For this review, take the finished solid that the model builds, in its own axes (mm). Coordinates: 2 decimals unless noted, no trailing zeros. Write each loop counter-clockwise with the first axis right and the second up, starting at its lowest first coordinate (ties: lowest second). Pieces come first, ordered by that corner, then holes. Notation, with made-up numbers: M 17.25,-37.5 L 69.25,-37.5 A32 cw 69.25,-3.5 Z; hole C -24.75,-32 d1. An arc over 180 degrees is marked long. One line per question, with ' | ' between items.
from build123d import *

# Parameters (mm, degrees)
F1_DEPTH  = 5
F0_W      = 115
F0_H      = 3
F0_W_2    = 3
F0_H_2    = 115
F2_DEPTH  = 2
F3_R      = 2.5
F4_DEPTH  = 5
F5_W      = 149
F5_H      = 149
F6_DEPTH  = 35
F7_R      = 1.5
F8_DEPTH  = 35
F9_W      = 149
F9_H      = 50.5775869712
F10_DEPTH = 200
F12_DEPTH = 2
F13_SIZE  = 1.99999


# Not quite as in the source:
# - a fillet or chamfer is up to 0.001 mm smaller than in the source, because OpenCascade refuses the exact size


with BuildPart() as f1:
    # F0 (on Top) → F1 (new body)
    with BuildSketch(Plane.XY):
        Polygon((74.5, 74.5), (60.5, 74.5), (-60.5, 74.5), (-74.5, 74.5), (-74.5, 60.5), (-74.5, -60.5), (-74.5, -74.5), (-60.5, -74.5), (60.5, -74.5), (74.5, -74.5), (74.5, -60.5), (74.5, 60.5), align=None)
        Polygon((57.5, 60.5), (60.5, 60.5), (60.5, 57.5), (60.5, -57.5), (60.5, -60.5), (57.5, -60.5), (-57.5, -60.5), (-60.5, -60.5), (-60.5, -57.5), (-60.5, 57.5), (-60.5, 60.5), (-57.5, 60.5), align=None, mode=Mode.SUBTRACT)
    extrude(amount=F1_DEPTH)

    # F0 (on Top) → F2 (join)
    with BuildSketch(Plane.XY):
        with Locations((0, 59)):
            Rectangle(F0_W, F0_H)
        with Locations((59, 59)):
            Rectangle(F0_W_2, F0_H)
        with Locations((59, 0)):
            Rectangle(F0_W_2, F0_H_2)
        with Locations((59, -59)):
            Rectangle(F0_W_2, F0_H)
        with Locations((0, -59)):
            Rectangle(F0_W, F0_H)
        with Locations((-59, 0)):
            Rectangle(F0_W_2, F0_H_2)
        with Locations((-59, -59)):
            Rectangle(F0_W_2, F0_H)
        with Locations((-59, 59)):
            Rectangle(F0_W_2, F0_H)
    extrude(amount=F2_DEPTH)

    # F3 (on face) → F4 (cut, through all)
    with BuildSketch(Plane.XY.offset(5)):
        with Locations((42.5219088793, 68.0854469538)):
            Circle(F3_R)
    extrude(amount=-F4_DEPTH, mode=Mode.SUBTRACT)

    # F5 (on face) → F6 (join)
    with BuildSketch(Plane.XY.offset(5)):
        Rectangle(F5_W, F5_H)
        Polygon((-60.5, 71.5), (60.5, 71.5), (71.5, 71.5), (71.5, 60.5), (71.5, -60.5), (71.5, -71.5), (60.5, -71.5), (-60.5, -71.5), (-71.5, -71.5), (-71.5, -60.5), (-71.5, 60.5), (-71.5, 71.5), align=None, mode=Mode.SUBTRACT)
    extrude(amount=F6_DEPTH)

    # F7 (on face) → F8 (join)
    with BuildSketch(Plane.XY.offset(40)):
        with BuildLine():
            ThreePointArc((-71.5, 64.975068144), (-66.8161183572, 65.4466893403), (-64.6000009775, 69.6000009775))
            ThreePointArc((-64.6000009775, 69.6000009775), (-64.6946638756, 70.5683335217), (-64.975068144, 71.5))
            Line((-64.975068144, 71.5), (-71.5, 71.5))
            Line((-71.5, 71.5), (-71.5, 64.975068144))
        make_face()
        with Locations((-69.6000009775, 69.6000009775)):
            Circle(F7_R, mode=Mode.SUBTRACT)
        with BuildLine():
            Line((71.5, 71.5), (64.975068144, 71.5))
            ThreePointArc((64.975068144, 71.5), (66.0644670716, 66.0644670716), (71.5, 64.975068144))
            Line((71.5, 64.975068144), (71.5, 71.5))
        make_face()
        with Locations((69.6000009775, 69.6000009775)):
            Circle(F7_R, mode=Mode.SUBTRACT)
        with BuildLine():
            Line((71.5, -71.5), (71.5, -64.975068144))
            ThreePointArc((71.5, -64.975068144), (66.0644670716, -66.0644670716), (64.975068144, -71.5))
            Line((64.975068144, -71.5), (71.5, -71.5))
        make_face()
        with Locations((69.6000009775, -69.6000009775)):
            Circle(F7_R, mode=Mode.SUBTRACT)
        with BuildLine():
            ThreePointArc((-64.6000009775, -69.6000009775), (-66.8161183572, -65.4466893403), (-71.5, -64.975068144))
            Line((-71.5, -64.975068144), (-71.5, -71.5))
            Line((-71.5, -71.5), (-64.975068144, -71.5))
            ThreePointArc((-64.975068144, -71.5), (-64.6946638756, -70.5683335217), (-64.6000009775, -69.6000009775))
        make_face()
        with Locations((-69.6000009775, -69.6000009775)):
            Circle(F7_R, mode=Mode.SUBTRACT)
    extrude(amount=-F8_DEPTH)

    # F9 (on face) → F10 (cut)
    with BuildSketch(Plane.XZ.offset(74.5)):
        with Locations((0, 12.7112065144)):
            Rectangle(F9_W, F9_H)
    extrude(amount=-F10_DEPTH, mode=Mode.SUBTRACT)

    # F11 (on face) → F12 (join)
    with BuildSketch(Plane.XY.offset(40)):
        with BuildLine():
            ThreePointArc((-64.975068144, 71.5), (-64.6974956073, 68.6174323567), (-66.0644670716, 66.0644670716))
            Line((-66.0644670716, 66.0644670716), (66.0644670716, 66.0644670716))
            ThreePointArc((66.0644670716, 66.0644670716), (64.6974956073, 68.6174323567), (64.975068144, 71.5))
            Line((64.975068144, 71.5), (-64.975068144, 71.5))
        make_face()
        with BuildLine():
            ThreePointArc((71.5, 64.975068144), (68.6174323567, 64.6974956073), (66.0644670716, 66.0644670716))
            Line((66.0644670716, 66.0644670716), (66.0644670716, -66.0644670716))
            ThreePointArc((66.0644670716, -66.0644670716), (68.6174323567, -64.6974956073), (71.5, -64.975068144))
            Line((71.5, -64.975068144), (71.5, 64.975068144))
        make_face()
        with BuildLine():
            Line((66.0644670716, -66.0644670716), (-66.0644670716, -66.0644670716))
            ThreePointArc((-66.0644670716, -66.0644670716), (-64.6974956073, -68.6174323567), (-64.975068144, -71.5))
            Line((-64.975068144, -71.5), (64.975068144, -71.5))
            ThreePointArc((64.975068144, -71.5), (64.6974956073, -68.6174323567), (66.0644670716, -66.0644670716))
        make_face()
        with BuildLine():
            Line((-66.0644670716, -66.0644670716), (-66.0644670716, 66.0644670716))
            ThreePointArc((-66.0644670716, 66.0644670716), (-68.6174323567, 64.6974956073), (-71.5, 64.975068144))
            Line((-71.5, 64.975068144), (-71.5, -64.975068144))
            ThreePointArc((-71.5, -64.975068144), (-68.6174323567, -64.6974956073), (-66.0644670716, -66.0644670716))
        make_face()
    extrude(amount=-F12_DEPTH)

    # F13 (size 2 in the source; OpenCascade refuses exactly that, so slightly less here)
    f13_edges = [f1.edges().sort_by_distance(p)[0] for p in [
        (-71.100001, 69.600001, 40),
        (68.100001, 69.600001, 40),
        (68.100001, -69.600001, 40),
        (-71.100001, -69.600001, 40),
    ]]
    chamfer(f13_edges, length=F13_SIZE)


solid = f1.part
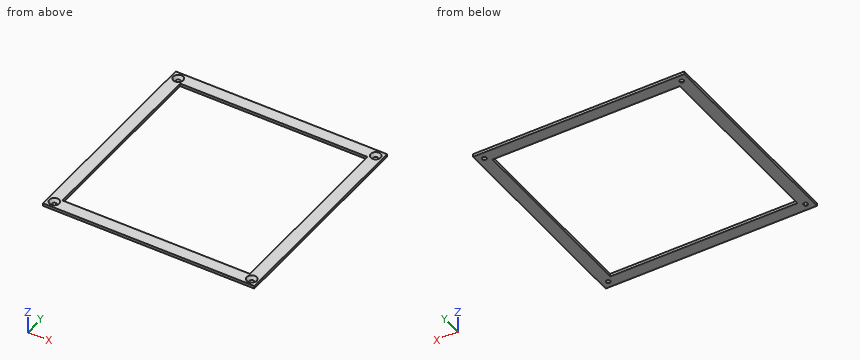
1. Take a section at A-A on y = 22.5. State the section outline as (x, z) points, plus the area to 3 significant figures.
Computed values:
outline: M -74.5,38 L -66.06,38 L -66.06,40 L -74.5,40 Z; M 66.06,38 L 74.5,38 L 74.5,40 L 66.06,40 Z | area: 33.7 mm2
2. For line 1 along Y through (x, z) = (-39.5, 38.9); line 2 along X through (y, z) = (-69.6, 38.05), list the stretches that pass through material, from the lowest coordinate up.
Computed values:
line 1: y = -74.5 to -66.06, 66.06 to 74.5 | line 2: x = -74.5 to -71.15, -68.05 to 68.05, 71.15 to 74.5
3. Take a section at C-C on z = 39.6. State the section outline as (x, y) points.
Computed values:
outline: M -74.5,-74.5 L 74.5,-74.5 L 74.5,74.5 L -74.5,74.5 Z; hole C -69.6,-69.6 d6.2; hole C -69.6,69.6 d6.2; hole M -66.06,-66.06 L 66.06,-66.06 L 66.06,66.06 L -66.06,66.06 Z; hole C 69.6,-69.6 d6.2; hole C 69.6,69.6 d6.2
